Design review of the part built by this model. Coordinates are the model's own, in mm. Round coordinates to 2 decimals unless told otherwise and drop trailing zeros. Order: outer loops, then holes, each group sorted by start corner. A loop starts at its lowest first (then second) coordinate and runs counter-clockwise, first axis right, second up.
from build123d import *

# Parameters (mm, degrees)
F0_W     = 130
F0_H     = 36.4172644913
F1_DEPTH = 5
F2_D     = 4.1
F3_D     = 5.4102


with BuildPart() as f1:
    # F0 (on Top) → F1 (new body)
    with BuildSketch(Plane.XY):
        with Locations((-1.3452520967, 18.2086322457)):
            Rectangle(F0_W, F0_H)
        with Locations((-1.3452520967, -18.2086322457)):
            Rectangle(F0_W, F0_H)
    extrude(amount=F1_DEPTH)

    # F2 (through all)
    with Locations(Plane(origin=(0, 0, 0), x_dir=(1, 0, 0), z_dir=(0, 0, -1))):
        with Locations((-61.3452520967, -30), (-61.3452520967, 30), (58.6547479033, -30), (58.6547479033, 30)):
            Hole(F2_D / 2)

    # F3 (through all)
    with Locations(Plane(origin=(0, 0, 0), x_dir=(1, 0, 0), z_dir=(0, 0, -1))):
        with Locations((0, 0)):
            Hole(F3_D / 2)


solid = f1.part
1) Take a section at C-C on y = 30. Give the boundary of the cut face in (x, z), plus the area to 3 significant figures.
Results:
outline: (-66.35, 0) - (-63.4, 0) - (-63.4, 5) - (-66.35, 5) - close; (-59.3, 0) - (56.6, 0) - (56.6, 5) - (-59.3, 5) - close; (60.7, 0) - (63.65, 0) - (63.65, 5) - (60.7, 5) - close
area: 609 mm2
2) Clearance check with a flat-ended pin moving along its axis: P1, Ø3.5, axis at x = 58.65, y = 30, coming from the -Z side. State where the tip first meets the part, or that it passes through.
Results:
P1: passes through
3) To check wall thickness, follow line 1 along X through (y, z) = (-30, 2.5); line 2 along Y through (x, z) = (58.5, 2.2); line 3 along X through (y, z) = (31.5, 4.55). State the ranges of each line that lie inside material, in increasing order.
Results:
line 1: x = -66.35 to -63.4, -59.3 to 56.6, 60.7 to 63.65
line 2: y = -36.42 to -32.04, -27.96 to 27.96, 32.04 to 36.42
line 3: x = -66.35 to -62.74, -59.95 to 57.26, 60.05 to 63.65
4) Take a section at A-A on x = 0. Give the boundary of the cut face in (y, z).
Results:
outline: (-36.42, 0) - (-2.71, 0) - (-2.71, 5) - (-36.42, 5) - close; (2.71, 0) - (36.42, 0) - (36.42, 5) - (2.71, 5) - close
5) Take a section at B-B on y = 0. Give the boundary of the cut face in (x, z), plus the area to 3 significant figures.
Results:
outline: (-66.35, 0) - (-2.71, 0) - (-2.71, 5) - (-66.35, 5) - close; (2.71, 0) - (63.65, 0) - (63.65, 5) - (2.71, 5) - close
area: 623 mm2
6) The part is to be moulded in two halves that separate along X. For faces 1 (the face through (-66.345, 1, 2)), 2 (the face through (-2, 9, 0)), 3 (the face through (-2.58, -0.81, 2.53)), say which applies: released by +X, released by -X, zero draft, split by the parting line, or undercut.
Results:
face 1: released by -X
face 2: zero draft
face 3: undercut
